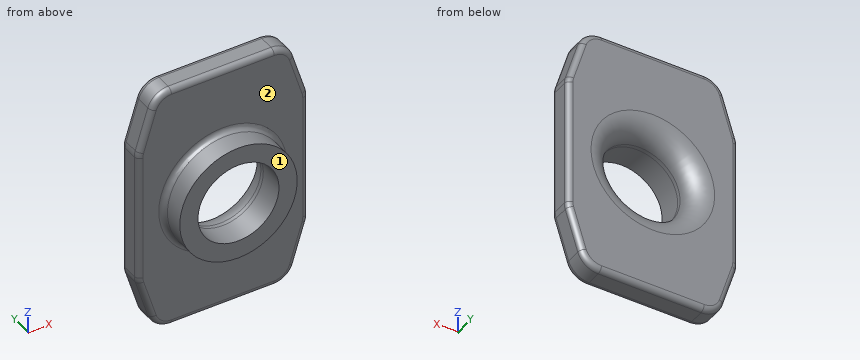
```python
from build123d import *

# Parameters (mm, degrees)
SKETCH1_R           = 2.413
BOSS_EXTRUDE1_DEPTH = 1.5
BOSS_EXTRUDE2_START = 1.5
SKETCH2_R           = 3.5
SKETCH2_R_2         = 2.413
BOSS_EXTRUDE2_DEPTH = 1.5
FILLET1_R           = 1.27
FILLET2_R           = 0.3175


with BuildPart() as part:
    # Sketch1 → Boss-Extrude1 (new body)
    with BuildSketch(Plane(origin=(0, 0, 0), x_dir=(1, 0, 0), z_dir=(0, 1, 0))):
        Polygon((4, 7.5), (-4, 7.5), (-5.08, 4), (-5.08, -4), (-4, -7.5), (4, -7.5), (5.08, -4), (5.08, 4), align=None)
        with Locations(Location((0, 0, 0), (0, 0, 270))):
            Circle(SKETCH1_R, mode=Mode.SUBTRACT)
    extrude(amount=BOSS_EXTRUDE1_DEPTH)

    # Sketch2 → Boss-Extrude2 (add)
    with BuildSketch(Plane.XZ.offset(BOSS_EXTRUDE2_START)):
        with Locations(Location((0, 0, 0), (0, 0, 90))):
            Circle(SKETCH2_R)
        with Locations(Location((0, 0, 0), (0, 0, 90))):
            Circle(SKETCH2_R_2, mode=Mode.SUBTRACT)
    extrude(amount=-BOSS_EXTRUDE2_DEPTH)

    # Fillet1
    fillet1_edges = [part.edges().sort_by_distance(p)[0] for p in [
        (-5.08, 0.75, 4),
        (-5.08, 0.75, -4),
        (-4, 0.75, -7.5),
        (4, 0.75, -7.5),
        (5.08, 0.75, -4),
        (5.08, 0.75, 4),
        (4, 0.75, 7.5),
        (-4, 0.75, 7.5),
        (0, 1.5, -2.413),
    ]]
    fillet(fillet1_edges, radius=FILLET1_R)

    # Fillet2
    fillet2_edges = [part.edges().sort_by_distance(p)[0] for p in [
        (0, 0, -3.5),
        (-4.64993803, 1.5, 5.393719347),
        (0, 1.5, 7.5),
        (4.64993803, 1.5, 5.393719347),
        (5.08, 1.5, 0),
        (4.64993803, 1.5, -5.393719347),
        (0, 1.5, -7.5),
        (-4.64993803, 1.5, -5.393719347),
        (-5.08, 1.5, 0),
        (5.065805445, 1.5, 3.997859771),
        (5.065805445, 1.5, -3.997859771),
        (3.816897156, 1.5, -7.251877837),
        (-3.816897156, 1.5, -7.251877837),
        (-5.065805445, 1.5, -3.997859771),
        (-5.065805445, 1.5, 3.997859771),
        (-3.816897156, 1.5, 7.251877837),
        (3.816897156, 1.5, 7.251877837),
        (4.64993803, 0, 5.393719347),
        (-4.64993803, 0, 5.393719347),
        (-5.08, 0, 0),
        (-4.64993803, 0, -5.393719347),
        (0, 0, -7.5),
        (4.64993803, 0, -5.393719347),
        (5.08, 0, 0),
        (0, 0, 7.5),
        (5.065805445, 0, 3.997859771),
        (5.065805445, 0, -3.997859771),
        (3.816897156, 0, -7.251877837),
        (-3.816897156, 0, -7.251877837),
        (-5.065805445, 0, -3.997859771),
        (-5.065805445, 0, 3.997859771),
        (-3.816897156, 0, 7.251877837),
        (3.816897156, 0, 7.251877837),
    ]]
    fillet(fillet2_edges, radius=FILLET2_R)


solid = part.part
```
Could you check a few things on this model? Use its own coordinates, in mm. Face numbers are marked on the shaded views. A direction names the side the tool comes from. Round coordinates to 2 decimals unless told otherwise and drop trailing zeros. Write each loop counter-clockwise with the first axis right and the second up, starting at its lowest first coordinate (ties: lowest second). Pieces come first, ordered by that corner, then holes.
(1) Suppose I cut it at C-C on y = 0.85. Write out the boundary of the cut face in (x, z).
Findings below:
outline: (-5.08, -3.81) arc R1.27 ccw to (-5.02, -4.18) - (-4.28, -6.6) arc R1.27 ccw to (-3.06, -7.5) - (3.06, -7.5) arc R1.27 ccw to (4.28, -6.6) - (5.02, -4.18) arc R1.27 ccw to (5.08, -3.81) - (5.08, 3.81) arc R1.27 ccw to (5.02, 4.18) - (4.28, 6.6) arc R1.27 ccw to (3.06, 7.5) - (-3.06, 7.5) arc R1.27 ccw to (-4.28, 6.6) - (-5.02, 4.18) arc R1.27 ccw to (-5.08, 3.81) - close; hole circle Ø5.15 at (0, 0)
(2) Suppose I cut it at D-D on y = -1.1. Write out the boundary of the cut face in (x, z).
Findings below:
outline: circle Ø7 at (0, 0); hole circle Ø4.83 at (0, 0)
(3) Which directions (+Z, -Z, +X, -X, +Y, -Y) give clear straight access to the entire face, cutting with the end or side of a thin tool? Please do the marked faces 1 and 2.
Findings below:
face 1: +Z, -Z, +X, -X, -Y
face 2: -Y
(4) Suppose I cut it at B-B on x = 0. Write out the boundary of the cut face in (y, z) (1 decimal).
Findings below:
outline: (-1.5, -3.5) - (-0.3, -3.5) arc R0.3 cw to (0, -3.8) - (0, -7.2) arc R0.3 ccw to (0.3, -7.5) - (1.2, -7.5) arc R0.3 ccw to (1.5, -7.2) - (1.5, -3.7) arc R1.3 ccw to (0.2, -2.4) - (-1.5, -2.4) - close; (-1.5, 2.4) - (0.2, 2.4) arc R1.3 ccw to (1.5, 3.7) - (1.5, 7.2) arc R0.3 ccw to (1.2, 7.5) - (0.3, 7.5) arc R0.3 ccw to (0, 7.2) - (0, 3.8) arc R0.3 cw to (-0.3, 3.5) - (-1.5, 3.5) - close
(5) Suppose I cut it at A-A on z = 0. Write out the boundary of the cut face in (x, y) (1 decimal), and give its area (3 significant figures).
Findings below:
outline: (-5.1, 0.3) arc R0.3 ccw to (-4.8, 0) - (-3.8, 0) arc R0.3 cw to (-3.5, -0.3) - (-3.5, -1.5) - (-2.4, -1.5) - (-2.4, 0.2) arc R1.3 ccw to (-3.7, 1.5) - (-4.8, 1.5) arc R0.3 ccw to (-5.1, 1.2) - close; (2.4, -1.5) - (3.5, -1.5) - (3.5, -0.3) arc R0.3 cw to (3.8, 0) - (4.8, 0) arc R0.3 ccw to (5.1, 0.3) - (5.1, 1.2) arc R0.3 ccw to (4.8, 1.5) - (3.7, 1.5) arc R1.3 ccw to (2.4, 0.2) - close
area: 10.5 mm2
(6) If I drill on probe 1 along X at (y, z) = (-1.2, 0); probe 2 along Y at (x, z) = (2.25, 6); probe 3 along X at (y, z) = (0.25, 0), over which ranges is the centre line in solid material (lowest first)?
Findings below:
probe 1: x = -3.5 to -2.41, 2.41 to 3.5
probe 2: y = 0 to 1.5
probe 3: x = -5.07 to -2.41, 2.41 to 5.07
